Work out the finished part from the listing and answer in its coordinate system (mm). Round coordinates to 2 decimals unless told otherwise and drop trailing zeros. Loops run counter-clockwise (first coordinate to the right, second up) from the corner with the lowest first, then second, coordinate; pieces in that order, holes last. Notation, with made-up numbers: M 32,47 L 40,47 A25 cw 40,82 Z; hole C -35,7.25 d7. An arc over 180 degrees is marked long. One line per item, written item: value.
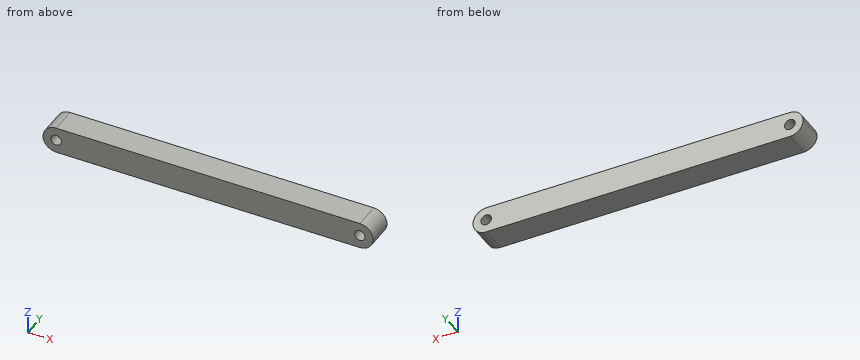
```python
from build123d import *

# Parameters (mm, degrees)
SKETCH_1_W          = 125
SKETCH_1_H          = 10
EXTRUDE_1_DEPTH     = 10
FILLET_1_R          = 5
SKETCH_2_R          = 2
CUT_EXTRUDE_1_DEPTH = 10


with BuildPart() as part:
    # 스케치1 → 보스-돌출1 (new body)
    with BuildSketch(Plane.XY):
        Rectangle(SKETCH_1_W, SKETCH_1_H)
    extrude(amount=EXTRUDE_1_DEPTH)

    # 필렛1
    fillet_1_edges = [part.edges().sort_by_distance(p)[0] for p in [
        (62.5, 0, 10),
        (62.5, 0, 0),
        (-62.5, 0, 0),
        (-62.5, 0, 10),
    ]]
    fillet(fillet_1_edges, radius=FILLET_1_R - 0.0001)  # a hair under: the kernel refuses the full size

    # 스케치2 → 컷-돌출1 (cut)
    with BuildSketch(Plane(origin=(0, 5, 0), x_dir=(1, 0, 0), z_dir=(0, 1, 0))):
        with Locations(Location((-57.5, -5, 0), (0, 0, 270))):
            Circle(SKETCH_2_R)
        with Locations(Location((57.5, -5, 0), (0, 0, 270))):
            Circle(SKETCH_2_R)
    extrude(amount=-CUT_EXTRUDE_1_DEPTH, mode=Mode.SUBTRACT)


solid = part.part
```
1) Find section A-A (y = -0.25). Give the number of separate pieces and of enclosed holes in the cut face, then the cut area to 3 significant figures.
Check values:
separate pieces: 1
enclosed holes: 2
area: 1,200 mm2
2) Find section B-B (z = 8.25). Give the vertices of the cut face in (x, y), then the cut area to 3 significant figures.
Check values:
outline: M -61.3,-5 L 61.3,-5 L 61.3,5 L -61.3,5 Z
area: 1,230 mm2
3) Find the intervals of material crossed by probe 1 along X at (y, z) = (-1, 5); probe 2 along X at (y, z) = (-3.5, 4); probe 3 along Z at (x, y) = (-56.5, 1.25), in increasing order. Write a range as from..to.
Check values:
probe 1: -62.5..-59.5, -55.5..55.5, 59.5..62.5
probe 2: -62.4..-59.23, -55.77..55.77, 59.23..62.4
probe 3: 0..3.27, 6.73..10
4) Each of these flat-tipped pins is pushed along its axis until it touches: pin 1 (2 mm diameter, centred on y = -3, z = 7.5, fed in from -X); pin 2 (5 mm diameter, centred on y = -1.5, z = 1.5, fed in from +X); pin 3 (2 mm diameter, centred on y = 1.5, z = 6.5, fed in from -X). Where does it stop, or does it pass through?
Check values:
pin 1: x = -62.27
pin 2: x = 62.4
pin 3: x = -62.47
